from build123d import *

# Parameters (mm, degrees)
SKETCH_1_R          = 1.9
EXTRUDE_1_DEPTH     = 69
SKETCH_2_R          = 2.5
CUT_EXTRUDE_1_DEPTH = 2.1


with BuildPart() as part:
    # 草图1 → 凸台-拉伸1 (new body)
    with BuildSketch(Plane(origin=(0, 0, 0), x_dir=(0, 0, -1), z_dir=(1, 0, 0))):
        with BuildLine():
            Line((0, 0), (19, 0))
            Line((19, 0), (19, -1.1))
            Line((19, -1.1), (0, -1.1))
            Line((0, -1.1), (-3, -1.1))
            ThreePointArc((-3, -1.1), (-4.284523258, 4.611088342), (-0.678362647, 0))
            Line((-0.678362647, 0), (0, 0))
        make_face()
        with Locations((-3, 1.9)):
            Circle(SKETCH_1_R, mode=Mode.SUBTRACT)
    extrude(amount=EXTRUDE_1_DEPTH)

    # 草图2 → 切除-拉伸1 (cut, through all)
    with BuildSketch(Plane(origin=(0, 0, 0), x_dir=(1, 0, 0), z_dir=(0, 1, 0))):
        with Locations((8.5, 9)):
            Circle(SKETCH_2_R)
        with Locations((60.5, 9)):
            Circle(SKETCH_2_R)
        with Locations((34.5, 11)):
            Circle(SKETCH_2_R)
    extrude(amount=-CUT_EXTRUDE_1_DEPTH, mode=Mode.SUBTRACT)


solid = part.part
CAD build for the part. Positions are in the model's coordinates, mm. Coordinates: 2 decimals unless noted, no trailing zeros. Write each loop counter-clockwise with the first axis right and the second up, starting at its lowest first coordinate (ties: lowest second). Pieces come first, ordered by that corner, then holes. Notation, with made-up numbers: M -19.5,66 L -0.5,66 A15 cw -0.5,73 Z; hole C 68.25,-11 d10. An arc over 180 degrees is marked long. Return JSON: item names as keys, results as strings.
Item 1: Slice it at B-B, the plane y = 1.9. Write the cut outline in (x, z).
Findings below:
{"outline": "M 0,0 L 69,0 L 69,1.1 L 0,1.1 Z; M 0,4.9 L 69,4.9 L 69,6 L 0,6 Z"}
Item 2: Two-plate mould, pull along X, no slides. Class faces 1 (the flat face through (0, -0.5, -3.8)), 2 (the flat face through (34, -1.1, -8)), 3 (the cylindrical face through (62.81, -0.54, -8.04)): +X half, -X half, draft (parallel to the pull), parting line (faces both ways), or undercut.
Findings below:
{"face 1": "-X half", "face 2": "draft", "face 3": "undercut"}
Item 3: Slice it at C-C, the plane x = 31. Write the cut outline in (y, z).
Findings below:
{"outline": "M -1.1,-19 L 0,-19 L 0,0.68 A3 ccw long -1.1,3 Z; hole C 1.9,3 d3.8"}
Item 4: Slice it at A-A, the plane x = 60.5. Write the cut outline in (y, z).
Findings below:
{"outline": "M -1.1,-19 L 0,-19 L 0,-11.5 L -1.1,-11.5 Z; M -1.1,-6.5 L 0,-6.5 L 0,0.68 A3 ccw long -1.1,3 Z; hole C 1.9,3 d3.8"}
Item 5: Probe line 1 (X direction, y = -0.9, z = -9); line 2 (Y direction, x = 38.5, z = 3); line 3 (Y direction, x = 50.5, z = -7). List the from-to ranges inside material, lowest first. Write a range as from..to.
Findings below:
{"line 1": "x = 0..6, 11..33, 36..58, 63..69", "line 2": "y = -1.1..0, 3.8..4.9", "line 3": "y = -1.1..0"}
Item 6: Drop flat-ended pins along their axis: pin 1 Ø4 at (x, z) = (60.5, -9) entering from -Y; pin 2 Ø6 at (x, z) = (46.5, -8) entering from +Y; pin 3 Ø2 at (x, y) = (59.5, 4) entering from +Z; pin 4 Ø1.5 at (x, y) = (34, 4) entering from +Z. Give the stop position or say it passes through.
Findings below:
{"pin 1": "passes through", "pin 2": "stops at y = 0", "pin 3": "stops at z = 5.79", "pin 4": "stops at z = 5.68"}
